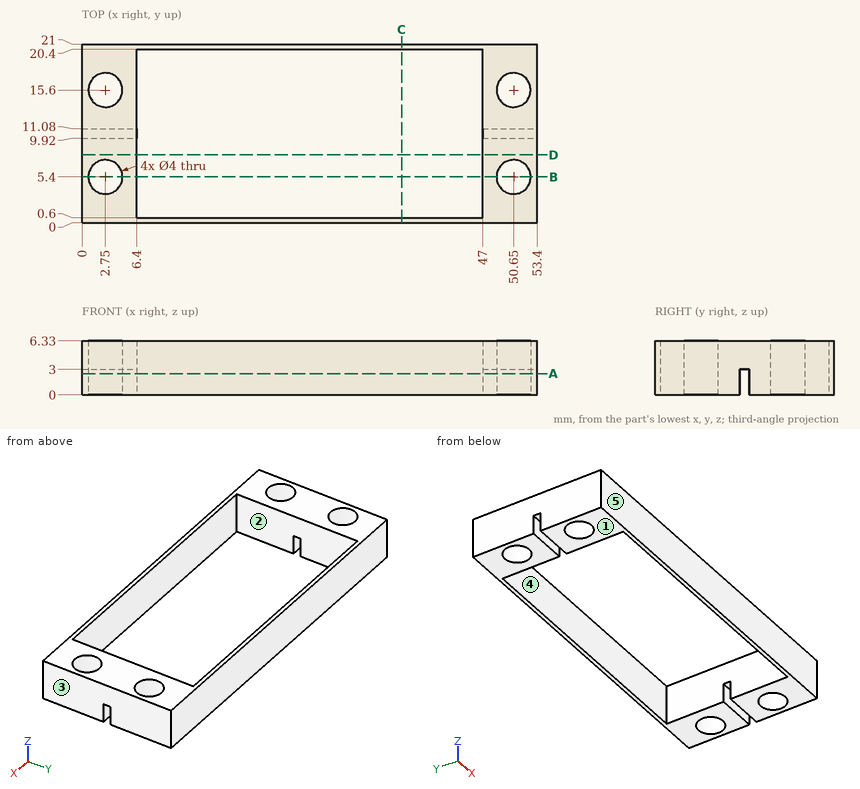
Part print with two shaded views. Sizes in mm from the minimum x, y, z corner. A direction names the side the tool comes from. Round coordinates to 2 decimals unless told otherwise and drop trailing zeros. Loops run counter-clockwise (first coordinate to the right, second up) from the corner with the lowest first, then second, coordinate; pieces in that order, holes last.
Item 1: Pin check, flat tip, straight feed: P1, Ø0.9, axis at x = 4, y = 10.5, coming from the -Z side. Stop position of the tip, or through.
Item 2: Saw through at D-D (y = 8). List the corners of the cut face in (x, z).
Item 3: Saw through at B-B (y = 5.4). List the corners of the cut face in (x, z).
Item 4: Two-plate mould, pull along X, no slides. Class the marked faces 1, 2 and 3: released by +X, released by -X, zero draft, split by the parting line, or undercut.
Item 5: Drill centre lines: line 1 along X through (y, z) = (15.5, 1.5); line 2 along Y through (x, z) = (2.75, 1.75); line 3 along Y through (x, z) = (50.65, 4). Where is each one in solid material? Low to high.
Item 6: Which spindle directions (+Z, -Z, +X, -X, +Y, -Y) get a long thin tool onto all of the face, cutting with end or side? Do the marked faces 4 and 5. Say none if no direction does.
Item 7: Saw through at A-A (z = 2.5). List the corners of the cut face in (x, y).
Item 8: Saw through at C-C (x = 37.5). List the corners of the cut face in (y, z), then the cut area to 3 significant figures.
Worked answers:
1. P1: stops at z = 3
2. outline: (0, 0) - (6.4, 0) - (6.4, 6.33) - (0, 6.33) - close; (47, 0) - (53.4, 0) - (53.4, 6.33) - (47, 6.33) - close
3. outline: (0, 0) - (0.75, 0) - (0.75, 6.33) - (0, 6.33) - close; (4.75, 0) - (6.4, 0) - (6.4, 6.33) - (4.75, 6.33) - close; (47, 0) - (48.65, 0) - (48.65, 6.33) - (47, 6.33) - close; (52.65, 0) - (53.4, 0) - (53.4, 6.33) - (52.65, 6.33) - close
4. face 1: zero draft
4. face 2: undercut
4. face 3: released by +X
5. line 1: x = 0 to 0.75, 4.75 to 6.4, 47 to 48.65, 52.65 to 53.4
5. line 2: y = 0 to 3.4, 7.4 to 9.92, 11.08 to 13.6, 17.6 to 21
5. line 3: y = 0 to 3.4, 7.4 to 13.6, 17.6 to 21
6. face 4: +Z, -Z
6. face 5: +Z, -Z, +X, -X, -Y
7. outline: (0, 0) - (53.4, 0) - (53.4, 9.92) - (47, 9.92) - (47, 0.6) - (6.4, 0.6) - (6.4, 9.92) - (0, 9.92) - close; (0, 11.08) - (6.4, 11.08) - (6.4, 20.4) - (47, 20.4) - (47, 11.08) - (53.4, 11.08) - (53.4, 21) - (0, 21) - close; hole circle Ø4 at (2.75, 5.4); hole circle Ø4 at (2.75, 15.6); hole circle Ø4 at (50.65, 5.4); hole circle Ø4 at (50.65, 15.6)
8. outline: (0, 0) - (0.6, 0) - (0.6, 6.33) - (0, 6.33) - close; (20.4, 0) - (21, 0) - (21, 6.33) - (20.4, 6.33) - close
8. area: 7.60 mm2
